from build123d import *

# Parameters (mm, degrees)
SKETCH12_W           = 75
SKETCH12_H           = 121.71
BOSS_EXTRUDE10_DEPTH = 12.7
SKETCH15_R           = 25.4
BOSS_EXTRUDE11_DEPTH = 15
SKETCH23_R           = 22.5
CUT_EXTRUDE7_DEPTH   = 186.429535576
FILLET2_R            = 12.8
SKETCH25_W           = 21.625
SKETCH25_H           = 12.7
CUT_EXTRUDE9_DEPTH   = 184.961470596
CUT_EXTRUDE10_DEPTH  = 184.961470596


with BuildPart() as part:
    # Sketch12 → Boss-Extrude10 (new body)
    with BuildSketch(Plane.XY):
        with Locations((99.625849364, 60.855)):
            Rectangle(SKETCH12_W, SKETCH12_H)
    extrude(amount=BOSS_EXTRUDE10_DEPTH)

    # Sketch15 → Boss-Extrude11 (add)
    with BuildSketch(Plane.XY.offset(12.7)):
        with Locations(Location((98.219620603, 38.627603634, 0), (0, 0, 180))):
            Circle(SKETCH15_R)
    extrude(amount=BOSS_EXTRUDE11_DEPTH)

    # Sketch23 → Cut-Extrude7 (cut, through all)
    with BuildSketch(Plane.XY.offset(27.7)):
        with Locations((98.219620603, 38.627603634)):
            Circle(SKETCH23_R)
    extrude(amount=-CUT_EXTRUDE7_DEPTH, mode=Mode.SUBTRACT)

    # Fillet2
    fillet2_edges = [part.edges().sort_by_distance(p)[0] for p in [
        (62.125849364, 0, 6.35),
        (137.125849364, 0, 6.35),
    ]]
    fillet(fillet2_edges, radius=FILLET2_R)

    # Sketch25 → Cut-Extrude9 (cut, through all)
    with BuildSketch(Plane.XY.offset(12.7)):
        with Locations((72.938349364, 115.36)):
            Rectangle(SKETCH25_W, SKETCH25_H)
        with Locations((126.313349364, 115.36)):
            Rectangle(SKETCH25_W, SKETCH25_H)
    extrude(amount=-CUT_EXTRUDE9_DEPTH, mode=Mode.SUBTRACT)

    # Sketch27 → Cut-Extrude10 (cut, through all)
    with BuildSketch(Plane.XY.offset(12.7)):
        Polygon((132.917349364, 109.01), (132.917349364, 104.311), (135.279349364, 104.311), (135.279349364, 98.469), (132.917349364, 98.469), (132.917349364, 93.77), (126.313349364, 93.77), (126.313349364, 98.469), (123.951349364, 98.469), (123.951349364, 104.311), (126.313349364, 104.311), (126.313349364, 109.01), align=None)
        Polygon((72.938349364, 98.469), (75.300349364, 98.469), (75.300349364, 104.311), (72.938349364, 104.311), (72.938349364, 109.01), (66.334349364, 109.01), (66.334349364, 104.311), (63.972349364, 104.311), (63.972349364, 98.469), (66.334349364, 98.469), (66.334349364, 93.77), (72.938349364, 93.77), align=None)
    extrude(amount=-CUT_EXTRUDE10_DEPTH, mode=Mode.SUBTRACT)


solid = part.part
Here's how the part is built. I have some questions about the finished solid (model axes, mm). A direction names the side the tool comes from. Coordinates: 2 decimals unless noted, no trailing zeros. Order: outer loops, then holes, each group sorted by start corner. A loop starts at its lowest first (then second) coordinate and runs counter-clockwise, first axis right, second up.
Item 1: For P1, Ø8, axis at y = 26, z = 21.5, coming from the +X side; P2, Ø5, axis at y = 82, z = 16, coming from the +X side; P3, Ø0.7, axis at x = 74, z = 7, coming from the -Y side; P4, Ø5.5, axis at x = 78, z = 6, coming from the +Y side, each with a flat end and sliding along its axis, tell me the tip position at first contact or that it passes through.
Result sheet:
P1: stops at x = 122.11
P2: passes through
P3: stops at y = 0.01
P4: stops at y = 109.01
Item 2: If we mould it in two halves opening along X, with no side actions, what happens to faces 4 (the face through (126.313, 96, 6)), 5 (the face through (83.751, 115, 6)), 6 (the face through (65, 98.469, 6)), 7 (the face through (78, 109.01, 6))? For each: +X half, -X half, draft (parallel to the pull), parting line (faces both ways), or undercut.
Result sheet:
face 4: undercut
face 5: -X half
face 6: undercut
face 7: draft
Item 3: If we section it at A-A on y = 102.5: List the corners of the cut face in (x, z) for me.
Result sheet:
outline: (62.13, 0) - (63.97, 0) - (63.97, 12.7) - (62.13, 12.7) - close; (75.3, 0) - (123.95, 0) - (123.95, 12.7) - (75.3, 12.7) - close; (135.28, 0) - (137.13, 0) - (137.13, 12.7) - (135.28, 12.7) - close
Item 4: For faces 1 (the face through (134, 104.311, 6)), 2 (the face through (64, 109.01, 6)), 3 (the face through (126.313, 107, 6)), which set-ups out of +Z, -Z, +X, -X, +Y, -Y let a thin tool reach every point of the face, with its end or its side?
Result sheet:
face 1: +Z, -Z
face 2: +Z, -Z, -X, +Y
face 3: +Z, -Z, +Y
Item 5: If we section it at B-B on x = 100: List the corners of the cut face in (y, z) for me, plus the area to 3 significant figures.
Result sheet:
outline: (0, 0) - (16.2, 0) - (16.2, 27.7) - (13.29, 27.7) - (13.29, 12.7) - (0, 12.7) - close; (61.06, 0) - (121.71, 0) - (121.71, 12.7) - (63.97, 12.7) - (63.97, 27.7) - (61.06, 27.7) - close
area: 1,060 mm2
Item 6: If we section it at D-D on y = 68: List the corners of the cut face in (x, z) for me.
Result sheet:
outline: (62.13, 0) - (137.13, 0) - (137.13, 12.7) - (62.13, 12.7) - close
Item 7: I need wall thicknesses on line 1 (X direction, y = 108, z = 6.5); line 2 (Y direction, x = 125, z = 11); line 3 (Y direction, x = 92, z = 10). Which ranges of each line are inside material? Lowest first, please.
Result sheet:
line 1: x = 62.13 to 66.33, 72.94 to 126.31, 132.92 to 137.13
line 2: y = 0.02 to 98.47, 104.31 to 109.01
line 3: y = 0 to 17, 60.25 to 121.71
Item 8: If we section it at C-C on y = 29: List the corners of the cut face in (x, z) for me.
Result sheet:
outline: (62.13, 0) - (77.88, 0) - (77.88, 27.7) - (74.71, 27.7) - (74.71, 12.7) - (62.13, 12.7) - close; (118.56, 0) - (137.13, 0) - (137.13, 12.7) - (121.72, 12.7) - (121.72, 27.7) - (118.56, 27.7) - close
